from build123d import *

# Parameters (mm, degrees)
SKETCH1_W                     = 57.912
SKETCH1_H                     = 49.8856
BOSS_EXTRUDE1_DEPTH           = 153.67
SHELL2_T                      = -2.54
SKETCH2_W                     = 52.832
SKETCH2_H                     = 44.8056
BOSS_EXTRUDE2_DEPTH           = 2.54
CUT_EXTRUDE1_REACH            = 166.139
BOSS_EXTRUDE3_DEPTH           = 2.54
SKETCH5_W                     = 34.7472
SKETCH5_H                     = 111.0742
BOSS_EXTRUDE4_DEPTH           = 2.1336
SKETCH6_R                     = 4.5212
BOSS_EXTRUDE5_DEPTH           = 9.2456
FILLET1_R                     = 1.27
CHAMFER1_SIZE                 = 0.762
FILLET2_R                     = 2.54
BOSS_EXTRUDE6_DEPTH           = 2.3114
CUT_EXTRUDE2_REACH            = 185.571
SKETCH8_R                     = 2.5
SKETCH9_R                     = 13.25
BOSS_EXTRUDE7_DEPTH           = 1.27
SKETCH10_R                    = 11.43
BOSS_EXTRUDE8_DEPTH           = 10.16
BOSS_EXTRUDE8_TAPER           = 10
SKETCH11_R                    = 11.43
BOSS_EXTRUDE9_DEPTH           = 6.096
BOSS_EXTRUDE9_DRAFT           = 10
BOSS_EXTRUDE9_PROFILE_2_DEPTH = 6.096
BOSS_EXTRUDE9_PROFILE_2_DRAFT = 10
CHAMFER2_SIZE                 = 1.905
CHAMFER2_SIZE_2               = 2.348489814
CHAMFER3_SIZE                 = 1.27


with BuildPart() as part:
    # Sketch1 → Boss-Extrude1 (new body)
    with BuildSketch(Plane(origin=(0, 0, 0), x_dir=(1, 0, 0), z_dir=(0, 1, 0))):
        Rectangle(SKETCH1_W, SKETCH1_H)
    extrude(amount=BOSS_EXTRUDE1_DEPTH)

    # Shell2
    shell2_openings = [part.faces().sort_by_distance(p)[0] for p in [
        (0, 153.67, 0),
    ]]
    offset(amount=SHELL2_T, openings=shell2_openings, kind=Kind.INTERSECTION)

    # Sketch2 → Boss-Extrude2 (add)
    with BuildSketch(Plane(origin=(0, 153.67, 0), x_dir=(1, 0, 0), z_dir=(0, 1, 0))):
        Rectangle(SKETCH2_W, SKETCH2_H)
    extrude(amount=-BOSS_EXTRUDE2_DEPTH)

    # Sketch3 → Cut-Extrude1 (cut, up to next)
    with BuildSketch(Plane.XY.offset(24.9428), mode=Mode.PRIVATE) as cut_extrude1_sk1:
        with BuildLine():
            Line((-16.51, 85.09), (-16.51, 125.73))
            ThreePointArc((-16.51, 125.73), (0, 142.24), (16.51, 125.73))
            Line((16.51, 125.73), (16.51, 85.09))
            ThreePointArc((16.51, 85.09), (0, 68.58), (-16.51, 85.09))
        make_face()
    cut_extrude1_tool1 = extrude(cut_extrude1_sk1.sketch, amount=-CUT_EXTRUDE1_REACH, mode=Mode.PRIVATE) & part.part
    add(cut_extrude1_tool1.solids().sort_by_distance((0, 105.41, 24.9428))[0], mode=Mode.SUBTRACT)

    # Sketch4 → Boss-Extrude3 (add)
    with BuildSketch(Plane(origin=(0, 0, 22.4028), x_dir=(-1, 0, 0), z_dir=(0, 0, -1))):
        with BuildLine():
            Line((19.05, 85.09), (19.05, 125.73))
            ThreePointArc((19.05, 125.73), (0, 144.78), (-19.05, 125.73))
            Line((-19.05, 125.73), (-19.05, 85.09))
            ThreePointArc((-19.05, 85.09), (0, 66.04), (19.05, 85.09))
        make_face()
    extrude(amount=BOSS_EXTRUDE3_DEPTH)

    # Sketch5 → Boss-Extrude4 (add)
    with BuildSketch(Plane(origin=(0, 0, -24.9428), x_dir=(-1, 0, 0), z_dir=(0, 0, -1))):
        with Locations((0, 41.9989)):
            Rectangle(SKETCH5_W, SKETCH5_H)
    extrude(amount=BOSS_EXTRUDE4_DEPTH)

    # Sketch6 → Boss-Extrude5 (add)
    with BuildSketch(Plane(origin=(0, 0, -27.0764), x_dir=(-1, 0, 0), z_dir=(0, 0, -1))):
        with Locations(Location((-11.0236, 91.186, 0), (0, 0, 180))):
            Circle(SKETCH6_R)
        with Locations(Location((-11.0236, 78.486, 0), (0, 0, 180))):
            Circle(SKETCH6_R)
        with Locations(Location((11.0236, 91.186, 0), (0, 0, 180))):
            Circle(SKETCH6_R)
        with Locations(Location((11.0236, 78.486, 0), (0, 0, 180))):
            Circle(SKETCH6_R)
    extrude(amount=BOSS_EXTRUDE5_DEPTH)

    # Fillet1
    fillet1_edges = [part.edges().sort_by_distance(p)[0] for p in [
        (6.5024, 91.186, -36.322),
        (6.5024, 78.486, -36.322),
        (-15.5448, 91.186, -36.322),
        (-15.5448, 78.486, -36.322),
    ]]
    fillet(fillet1_edges, radius=FILLET1_R)

    # Chamfer1
    chamfer1_edges = [part.edges().sort_by_distance(p)[0] for p in [
        (6.5024, 91.186, -27.0764),
        (6.5024, 78.486, -27.0764),
        (-15.5448, 91.186, -27.0764),
        (-15.5448, 78.486, -27.0764),
    ]]
    chamfer(chamfer1_edges, length=CHAMFER1_SIZE)

    # Fillet2
    fillet2_edges = [part.edges().sort_by_distance(p)[0] for p in [
        (28.956, 76.835, 24.9428),
        (-28.956, 76.835, 24.9428),
        (-28.956, 76.835, -24.9428),
        (28.956, 76.835, -24.9428),
    ]]
    fillet(fillet2_edges, radius=FILLET2_R)

    # Sketch7 → Boss-Extrude6 (add)
    with BuildSketch(Plane.XZ.offset(13.5382)):
        with BuildLine():
            Line((1.27, -8.0264), (59.0804, -8.0264))
            ThreePointArc((59.0804, -8.0264), (59.978425612, -8.398374388), (60.3504, -9.2964))
            Line((60.3504, -9.2964), (60.3504, -26.4414))
            ThreePointArc((60.3504, -26.4414), (60.164412806, -26.890412806), (59.7154, -27.0764))
            Line((59.7154, -27.0764), (53.3654, -27.0764))
            ThreePointArc((53.3654, -27.0764), (52.916387194, -26.890412806), (52.7304, -26.4414))
            Line((52.7304, -26.4414), (52.7304, -25.779323164))
            ThreePointArc((52.7304, -25.779323164), (52.682063503, -25.536319184), (52.544412806, -25.330310358))
            Line((52.544412806, -25.330310358), (43.096451224, -15.882348776))
            ThreePointArc((43.096451224, -15.882348776), (42.272415918, -15.331745987), (41.3004, -15.1384))
            Line((41.3004, -15.1384), (18.6436, -15.1384))
            ThreePointArc((18.6436, -15.1384), (17.745574388, -15.510374388), (17.3736, -16.4084))
            Line((17.3736, -16.4084), (17.3736, -27.0764))
            Line((17.3736, -27.0764), (-17.3736, -27.0764))
            Line((-17.3736, -27.0764), (-17.3736, -16.4084))
            ThreePointArc((-17.3736, -16.4084), (-17.745574388, -15.510374388), (-18.6436, -15.1384))
            Line((-18.6436, -15.1384), (-41.3004, -15.1384))
            ThreePointArc((-41.3004, -15.1384), (-42.272415918, -15.331745987), (-43.096451224, -15.882348776))
            Line((-43.096451224, -15.882348776), (-52.544412806, -25.330310358))
            ThreePointArc((-52.544412806, -25.330310358), (-52.682063503, -25.536319184), (-52.7304, -25.779323164))
            Line((-52.7304, -25.779323164), (-52.7304, -26.4414))
            ThreePointArc((-52.7304, -26.4414), (-52.916387194, -26.890412806), (-53.3654, -27.0764))
            Line((-53.3654, -27.0764), (-59.7154, -27.0764))
            ThreePointArc((-59.7154, -27.0764), (-60.164412806, -26.890412806), (-60.3504, -26.4414))
            Line((-60.3504, -26.4414), (-60.3504, -9.2964))
            ThreePointArc((-60.3504, -9.2964), (-59.978425612, -8.398374388), (-59.0804, -8.0264))
            Line((-59.0804, -8.0264), (-1.27, -8.0264))
            ThreePointArc((-1.27, -8.0264), (-0.371974388, -8.398374388), (0, -9.2964))
            ThreePointArc((0, -9.2964), (0.371974388, -8.398374388), (1.27, -8.0264))
        make_face()
    extrude(amount=BOSS_EXTRUDE6_DEPTH)

    # Sketch8 → Cut-Extrude2 (cut, up to next)
    with BuildSketch(Plane.XZ.offset(15.8496), mode=Mode.PRIVATE) as cut_extrude2_sk1:
        with Locations(Location((-52.5, -15.5264, 0), (0, 0, 270))):
            Circle(SKETCH8_R)
    cut_extrude2_tool1 = extrude(cut_extrude2_sk1.sketch, amount=-CUT_EXTRUDE2_REACH, mode=Mode.PRIVATE) & part.part
    # Sketch8 → Cut-Extrude2 (cut, up to next)
    with BuildSketch(Plane.XZ.offset(15.8496), mode=Mode.PRIVATE) as cut_extrude2_sk2:
        with Locations(Location((52.5, -15.5264, 0), (0, 0, 270))):
            Circle(SKETCH8_R)
    cut_extrude2_tool2 = extrude(cut_extrude2_sk2.sketch, amount=-CUT_EXTRUDE2_REACH, mode=Mode.PRIVATE) & part.part
    add(cut_extrude2_tool1.solids().sort_by_distance((-52.5, -15.8496, -15.5264))[0], mode=Mode.SUBTRACT)
    add(cut_extrude2_tool2.solids().sort_by_distance((52.5, -15.8496, -15.5264))[0], mode=Mode.SUBTRACT)

    # Sketch9 → Boss-Extrude7 (add)
    with BuildSketch(Plane(origin=(0, 153.67, 0), x_dir=(1, 0, 0), z_dir=(0, 1, 0))):
        with Locations(Location((0, 0, 0), (0, 0, 90))):
            Circle(SKETCH9_R)
    extrude(amount=BOSS_EXTRUDE7_DEPTH)

    # Sketch10 → Boss-Extrude8 (add)
    with BuildSketch(Plane(origin=(28.956, 0, 0), x_dir=(0, 0, -1), z_dir=(1, 0, 0))):
        with Locations((6.6548, 127.254)):
            Circle(SKETCH10_R)
    extrude(amount=BOSS_EXTRUDE8_DEPTH, taper=BOSS_EXTRUDE8_TAPER)


with BuildPart() as boss_extrude9_tool:
    # Sketch11 → Boss-Extrude9 (with draft: the straight prism first)
    with BuildSketch(Plane.ZY.offset(28.956)):
        with Locations((-7.1628, 127.508)):
            Circle(SKETCH11_R)
    extrude(amount=BOSS_EXTRUDE9_DEPTH)
    # Boss-Extrude9: the draft: its side faces are tilted about the plane it starts from
    boss_extrude9_sides = [boss_extrude9_tool.faces().sort_by_distance(p)[0] for p in [
        (-32.004, 127.508, -18.5928),
    ]]
    draft(boss_extrude9_sides, Plane.ZY.offset(28.956), BOSS_EXTRUDE9_DRAFT)


with BuildPart() as part_1:
    add(part.part)

    # Boss-Extrude9: add boss_extrude9_tool
    add(boss_extrude9_tool.part)


with BuildPart() as boss_extrude9_profile_2_tool:
    # Sketch11 → Boss-Extrude9 profile 2 (with draft: the straight prism first)
    with BuildSketch(Plane.ZY.offset(28.956)):
        with Locations((-7.1628, 71.628)):
            Circle(SKETCH11_R)
    extrude(amount=BOSS_EXTRUDE9_PROFILE_2_DEPTH)
    # Boss-Extrude9 profile 2: the draft: its side faces are tilted about the plane it starts from
    boss_extrude9_profile_2_sides = [boss_extrude9_profile_2_tool.faces().sort_by_distance(p)[0] for p in [
        (-32.004, 71.628, -18.5928),
    ]]
    draft(boss_extrude9_profile_2_sides, Plane.ZY.offset(28.956), BOSS_EXTRUDE9_PROFILE_2_DRAFT)


with BuildPart() as part_2:
    add(part_1.part)

    # Boss-Extrude9 profile 2: add boss_extrude9_profile_2_tool
    add(boss_extrude9_profile_2_tool.part)

    # Chamfer2
    # the kernel refuses this chamfer: 2.348489814, 1.905 mm, written as the material it takes off along each edge
    with BuildSketch(Plane(origin=(39.116, 127.254, -6.6548), x_dir=(0, 0, -1), z_dir=(0, 1, 0))) as chamfer2_piece_1:
        Polygon((9.638517876 + CHAMFER2_SIZE * 0.173648177667, CHAMFER2_SIZE * 0.984807753012), (9.638517876 - CHAMFER2_SIZE_2, 0), (9.638517876, 0), align=None)
    revolve(axis=Axis((39.116, 127.254, -6.6548), (-1, 0, 0)), mode=Mode.SUBTRACT)
    with BuildSketch(Plane(origin=(-35.052, 127.508, -7.1628), x_dir=(0, 0, 1), z_dir=(0, -1, 0))) as chamfer2_piece_2:
        Polygon((10.355110726 + CHAMFER2_SIZE * 0.173648177667, -CHAMFER2_SIZE * 0.984807753012), (10.355110726 - CHAMFER2_SIZE_2, 0), (10.355110726, 0), align=None)
    revolve(axis=Axis((-35.052, 127.508, -7.1628), (-1, 0, 0)), mode=Mode.SUBTRACT)
    with BuildSketch(Plane(origin=(-35.052, 71.628, -7.1628), x_dir=(0, 0, 1), z_dir=(0, -1, 0))) as chamfer2_piece_3:
        Polygon((10.355110726 + CHAMFER2_SIZE * 0.173648177667, -CHAMFER2_SIZE * 0.984807753012), (10.355110726 - CHAMFER2_SIZE_2, 0), (10.355110726, 0), align=None)
    revolve(axis=Axis((-35.052, 71.628, -7.1628), (-1, 0, 0)), mode=Mode.SUBTRACT)

    # Chamfer3
    chamfer3_edges = [part_2.edges().sort_by_distance(p)[0] for p in [
        (0, 68.58, 24.9428),
        (16.51, 105.41, 24.9428),
        (0, 142.24, 24.9428),
        (-16.51, 105.41, 24.9428),
    ]]
    chamfer(chamfer3_edges, length=CHAMFER3_SIZE)


solid = part_2.part
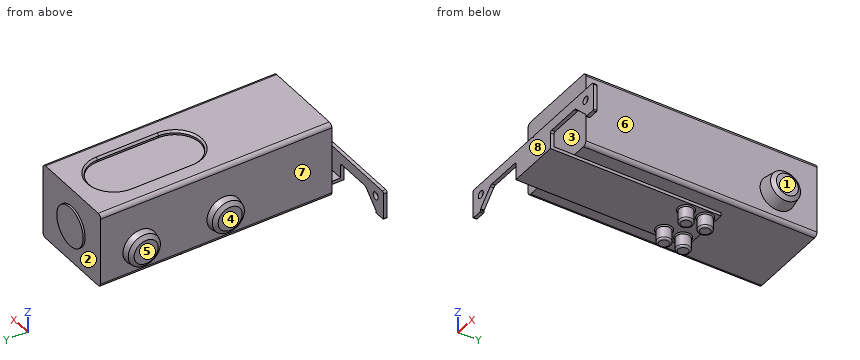
Read the model definition and answer for the solid it produces. Units are mm, in the model's axes. Face numbers are marked on the shaded views. A direction names the side the tool comes from. Round coordinates to 2 decimals unless told otherwise and drop trailing zeros. Order: outer loops, then holes, each group sorted by start corner. A loop starts at its lowest first (then second) coordinate and runs counter-clockwise, first axis right, second up. Notation, with made-up numbers: (22, 55) - (80, 55) arc R24 cw to (80, 79) - close; hole circle Ø2 at (33.5, 71). An arc over 180 degrees is marked (long way). Use one line per item in the form item = value. Start each with the question number.
(1) The part is cut by section C-C (z = 9). Give the vertices of the cut face in (x, y), then the cut area to 3 significant figures.
(2) For the marked faces 1, 2, 3 and 4, determine the directions among +Z, -Z, +X, -X, +Y, -Y from which every point of the face is accessible in a straight line to the end or side of a thin tool.
(3) Flat-ended cylindrical pins translate along their axes: pin 1 Ø3 at (y, z) = (96.5, 21) entering from -X; pin 2 Ø3 at (x, y) = (29.5, 56.5) entering from -Z; pin 3 Ø1 at (y, z) = (107, 23) entering from +X; pin 4 Ø4 at (x, z) = (31, -8) entering from -Y. Find the tip coordinate at first contact, or state that the pin passes through.
(4) The part is cut by section B-B (y = 11). Give the vertices of the cut face in (x, z).
(5) Find the intervals of material crossed by line 1 along Y through (x, z) = (24, -6); line 2 along Z through (x, y) = (-20, 77); line 3 along X through (y, z) = (144.5, -6), in increasing order. Write a range as from..to.
(6) The part is cut by section A-A (z = 18). Give the vertices of the cut face in (x, y), then the cut area to 3 significant figures.
(7) Determine the mould class of the marked faces 5, 6, 7 and 8 for opening direction Y: +Y half, -Y half, draft (parallel to the pull), parting line (faces both ways), or undercut.
Checked values:
q1.outline = (-28.96, 0) - (28.96, 0) - (28.96, 153.67) - (9.72, 153.67) - (9.72, 154.94) - (-9.72, 154.94) - (-9.72, 153.67) - (-28.96, 153.67) - close; hole (-26.42, 2.54) - (26.42, 2.54) - (26.42, 151.13) - (-26.42, 151.13) - close
q1.area = 1,070 mm^2
q2.face_1 = +Z, -Z, +X, +Y
q2.face_2 = +Y
q2.face_3 = +Z, +X, -X
q2.face_4 = +Z, -Z, -X, +Y
q3.pin_1 = -28.96
q3.pin_2 = -24.39
q3.pin_3 = 28.95
q3.pin_4 = -15.85
q4.outline = (-28.96, -22.4) arc R2.54 ccw to (-26.42, -24.94) - (-17.37, -24.94) - (-17.37, -27.08) - (17.37, -27.08) - (17.37, -24.94) - (26.42, -24.94) arc R2.54 ccw to (28.96, -22.4) - (28.96, 22.4) arc R2.54 ccw to (26.42, 24.94) - (-26.42, 24.94) arc R2.54 ccw to (-28.96, 22.4) - close; hole (-26.42, -22.4) - (26.42, -22.4) - (26.42, 22.4) - (-26.42, 22.4) - close
q5.line_1 = 0..2.54, 151.13..153.67
q5.line_2 = -24.94..-22.4, 22.4..24.94
q5.line_3 = -28.96..-26.42, 26.42..28.96
q6.outline = (-28.96, 0) - (28.96, 0) - (28.96, 153.67) - (-28.96, 153.67) - close; hole (-26.42, 2.54) - (26.42, 2.54) - (26.42, 151.13) - (-26.42, 151.13) - close
q6.area = 1,050 mm^2
q7.face_5 = draft
q7.face_6 = undercut
q7.face_7 = undercut
q7.face_8 = -Y half
